For this review, take the finished solid that the model builds, in its own axes (mm). Give positions to 0.01 mm unless a question says otherwise; leave off trailing zeros. Order: outer loops, then holes, each group sorted by start corner. A loop starts at its lowest first (then second) coordinate and runs counter-clockwise, first axis right, second up.
Item 1: For P1, Ø8, axis at x = -15, z = -45, coming from the +Y side; P2, Ø2.5, axis at x = -14.5, z = 46.5, coming from the +Y side, all flat-tipped, find the tip position at first contact; note any pin that passes through.
Item 2: For probe 1 along Z at (x, y) = (-15, 21); probe 2 along X at (y, z) = (-3, 14.5); probe 3 along Z at (x, y) = (-12.5, 19), list the stretches that pass through material, from the lowest coordinate up.
Item 3: Consider section A-A (z = 13.5). Give the boundary of the cut face in (x, y).
Item 4: Consider section C-C (y = 2.5). Give the boundary of the cut face in (x, z), plus the area to 3 significant figures.
Item 5: Consider section B-B (y = -17.5). Give the boundary of the cut face in (x, z).
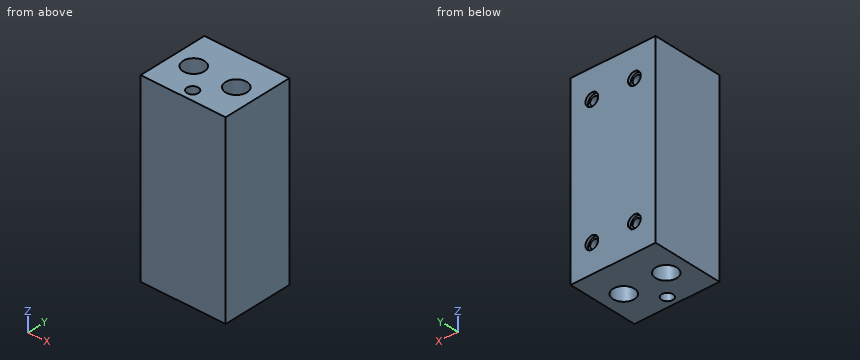
```python
from build123d import *

# Parameters (mm, degrees)
F0_W           = 60
F0_H           = 130
F1_DEPTH       = 25
F2_R           = 7.5
F2_R_2         = 4
F3_DEPTH       = 130.001
F5_D           = 6
F5_DEPTH       = 10
F5_CBORE_D     = 9
F5_CBORE_DEPTH = 2
F5_TIP         = 1.8025818571


with BuildPart() as f1:
    # F0 (on Front) → F1 (new body, symmetric)
    with BuildSketch(Plane.XZ):
        Rectangle(F0_W, F0_H)
    extrude(amount=F1_DEPTH, both=True)

    # F2 (on face) → F3 (cut, through all)
    with BuildSketch(Plane.XY.offset(65)):
        with Locations((-15, 0)):
            Circle(F2_R)
        with Locations((15, 0)):
            Circle(F2_R)
        with Locations((0, -17.5)):
            Circle(F2_R_2)
    extrude(amount=-F3_DEPTH, mode=Mode.SUBTRACT)

    # F5
    with Locations(Plane(origin=(0, 25, 0), x_dir=(-1, 0, 0), z_dir=(0, 1, 0))):
        with Locations((-15, 45), (15, 45), (15, -45), (-15, -45)):
            CounterBoreHole(F5_D / 2, F5_CBORE_D / 2, F5_CBORE_DEPTH, depth=F5_DEPTH)
            with Locations((0, 0, -(F5_DEPTH + F5_TIP / 2))):  # 118° drill point
                Cone(0, F5_D / 2, F5_TIP, mode=Mode.SUBTRACT)


solid = f1.part
```
Resolved:
1. P1: stops at y = 23
1. P2: stops at y = 14.9
2. probe 1: z = -65 to -48, -42 to 42, 48 to 65
2. probe 2: x = -30 to -21.87, -8.13 to 8.13, 21.87 to 30
2. probe 3: z = -65 to -46.66, -43.34 to 43.34, 46.66 to 65
3. outline: (-30, -25) - (30, -25) - (30, 25) - (-30, 25) - close; hole circle Ø15 at (-15, 0); hole circle Ø8 at (0, -17.5); hole circle Ø15 at (15, 0)
4. outline: (-30, -65) - (-22.07, -65) - (-22.07, 65) - (-30, 65) - close; (-7.93, -65) - (7.93, -65) - (7.93, 65) - (-7.93, 65) - close; (22.07, -65) - (30, -65) - (30, 65) - (22.07, 65) - close
4. area: 4,120 mm2
5. outline: (-30, -65) - (-4, -65) - (-4, 65) - (-30, 65) - close; (4, -65) - (30, -65) - (30, 65) - (4, 65) - close
